Check sheet for the modelled part. Datum: model origin and axes. Units: mm. A direction names the side the tool comes from. Coordinates: 2 decimals unless noted, no trailing zeros. Loops run counter-clockwise (first coordinate to the right, second up) from the corner with the lowest first, then second, coordinate; pieces in that order, holes last. Notation, with made-up numbers: (-19.75, -14) - (31.25, -14) arc R24 cw to (31.25, 12) - close; hole circle Ø6 at (-25, -10.75). An arc over 180 degrees is marked (long way). Write each question's results on one line, items separated by ' | '. Start each with the question number.
1. Thickness scan on line 1 (X direction, y = 1, z = -11); line 2 (Y direction, x = 16, z = 6.55); line 3 (X direction, y = 7, z = 0). Record the ranges inside material, lowest first. Write a range as [from, to].
2. Cross-section at C-C (z = -0.75). Record the cut outline in (x, y).
3. Tool access check on faces 4 (the face through (-6, 5, 3)), 5 (the face through (6, 5, 2)), 6 (the face through (-2.99, 3.45, -9.06)), 7 (the face through (-2, 5, -6)), 8 (the face through (-4, 5, -6)). Record the directions out of +Z, -Z, +X, -X, +Y, -Y that give a thin tool (end or side, any length) a straight path to the whole face; none if there is none.
4. Cross-section at D-D (y = 8.5). Record the cut outline in (x, z), and give its area (3 significant figures).
5. Draft check along X on faces 1 (the face through (17, 3, 6)), 2 (the face through (18, 5, 6)), 3 (the face through (3, 5, -11.75)). Enter one of: released by +X, released by -X, zero draft, split by the parting line, or undercut.
6. Cross-section at B-B (y = 5). Record the cut outline in (x, z).
7. Cross-section at A-A (x = 7). Record the cut outline in (y, z).
8. Gauge pin test, flat ends, axial feed: P1, Ø2.5, axis at y = 3, z = -9.5, coming from the +X side; P2, Ø3, axis at x = 14, y = 4, coming from the -Z side; P3, Ø3.5, axis at y = 4.5, z = 2, coming from the +X side. Record the tip position at first contact, or that the pin passes through.
Autodesk Inventor part; units mm, degrees
ref_plane "YZ Plane" through (0, 0, 0) normal (1, 0, 0) x (0, 1, 0)
ref_plane "XZ Plane" through (0, 0, 0) normal (0, 1, 0) x (-1, 0, 0)
ref_plane "XY Plane" through (0, 0, 0) normal (0, 0, 1) x (1, 0, 0)
sketch "Sketch1" plane through (0, 0, 0) normal (0, 1, 0) x (-1, 0, 0)
  circle A0 centre (0, 0) radius 4.25
  circle A1 centre (0, 0) radius 6
  line L0 (6, 0) -> (-6, 0)
  line L1 (-6, 0) -> (-6, 8.25)
  line L2 (-6, 8.25) -> (6, 8.25)
  line L3 (6, 8.25) -> (6, 0)
  line L4 (6, 8.25) -> (-18, 8.25)
  line L5 (-18, 8.25) -> (-18, 4.25)
  line L6 (-18, 4.25) -> (6, 4.25)
  line L7 (6, 4.25) -> (6, 8.25)
  point P0 (-4.2353, 4.25)
  point P1 (4.2353, 4.25)
  point P2 (6, 8.25)
  point P3 (-6, 4.25)
  point P4 (6, 4.25)
  dimension "d1" = 12
  dimension "d0" = 8.5
  dimension "d2" = 4
  dimension "d3" = 6
  dimension "d4" = 18
extrude "Extrusion1" add sketch "Sketch1" along normal blind 10 contours L0 A1 A0 | A0 L6 A1 L0 | A0 L0 A1 L6 | L6 A1 | A1 L6 L3 | L6 L1 L2 L3 A1 | A1 L1 L6 | L6 L5 L4 L1
sketch "Sketch2" plane through (0, 10, 0) normal (0, 1, 0) x (1, 0, 0)
  line L0 (-2, 1.8795) -> (2, 1.8795)
  line L1 (2, 1.8795) -> (2, 9.0075)
  line L2 (2, 9.0075) -> (-2, 9.0075)
  line L3 (-2, 9.0075) -> (-2, 1.8795)
  point P0 (0, 0)
  dimension "d7" = 2
  dimension "d8" = 2
extrude "Extrusion2" cut sketch "Sketch2" against normal blind 10
sketch "Sketch3" plane through (0, 10, 0) normal (0, 1, 0) x (1, 0, 0)
  line L0 (2, 3.75) -> (2, 5.6569)
  line L1 (2, 3.75) -> (4, 3.75)
  line L2 (4, 3.75) -> (4, 11.75)
  line L3 (4, 11.75) -> (2, 11.75)
  line L4 (2, 11.75) -> (2, 3.75)
  line L5 (-2, 3.75) -> (-2, 5.6569)
  line L6 (-2, 3.75) -> (-4, 3.75)
  line L7 (-4, 3.75) -> (-4, 11.75)
  line L8 (-4, 11.75) -> (-2, 11.75)
  line L9 (-2, 11.75) -> (-2, 3.75)
  point P0 (0, 0)
  dimension "d11" = 2
  dimension "d12" = 2
  dimension "d13" = 8
  dimension "d14" = 8
extrude "Extrusion3" add sketch "Sketch3" against normal blind 10
sketch "Sketch4" plane through (4, 10, -4.4721) normal (1, 0, 0) x (0, 0, -1)
  circle A0 centre (3.7779, -5) radius 1.75
  line L0 (7.2779, 0) -> (7.2779, -10)
  point P0 (-4.4721, -10)
  dimension "d17" = 3.5
  dimension "d18" = 3.5
extrude "Extrusion4" cut sketch "Sketch4" against normal through all
sketch "Sketch5" plane through (-6, 0, 8.25) normal (0, 0, 1) x (1, 0, 0)
  circle A0 centre (13, 3) radius 1
  circle A1 centre (22, 3) radius 1
  line L0 (0, 0) -> (0, 10)
  line L1 (0, 10) -> (24, 10)
  point P0 (6, 0)
  dimension "d21" = 2
  dimension "d22" = 9
  dimension "d24" = 7
  dimension "d27" = 16
extrude "Extrusion5" cut sketch "Sketch5" against normal through all
fillet "Fillet1" radius 2 1 edges at (-6, 5, 8.25)
properties part number "zstop"
Established:
1) line 1: [-4, -2], [2, 4] | line 2: [0, 2], [4, 10] | line 3: [-6, -4.25], [4.25, 6]
2) outline: (-5.95, 0) - (-4.18, 0) - (-4.18, 10) - (-5.95, 10) - close; (4.18, 0) - (5.95, 0) - (5.95, 10) - (4.18, 10) - close
3) face 4: +Z, -Z, -X, +Y, -Y | face 5: -Z, +X, +Y, -Y | face 6: +X, -X | face 7: -Z, +Y, -Y | face 8: -Z, -X, +Y, -Y
4) outline: (-6, 0) arc R6 ccw to (-4, -4.47) - (-4, -11.75) - (-2, -11.75) - (-2, -3.75) arc R4.25 cw (long way) to (2, -3.75) - (2, -11.75) - (4, -11.75) - (4, -4.47) arc R6 ccw to (6, 0) - (6, 4.25) - (18, 4.25) - (18, 8.25) - (-4, 8.25) arc R2 ccw to (-6, 6.25) - close | area: 165 mm^2
5) face 1: undercut | face 2: released by +X | face 3: zero draft
6) outline: (-6, 0) arc R6 ccw to (-4, -4.47) - (-4, -6.5) - (-2, -6.5) - (-2, -3.75) arc R4.25 cw (long way) to (2, -3.75) - (2, -6.5) - (4, -6.5) - (4, -4.47) arc R6 ccw to (6, 0) - (6, 4.25) - (18, 4.25) - (18, 8.25) - (-4, 8.25) arc R2 ccw to (-6, 6.25) - close; (-4, -11.75) - (-2, -11.75) - (-2, -10) - (-4, -10) - close; (2, -11.75) - (4, -11.75) - (4, -10) - (2, -10) - close
7) outline: (0, 4.25) - (2, 4.25) - (2, 8.25) - (0, 8.25) - close; (4, 4.25) - (10, 4.25) - (10, 8.25) - (4, 8.25) - close
8) P1: x = 4 | P2: z = 4.25 | P3: x = 6
